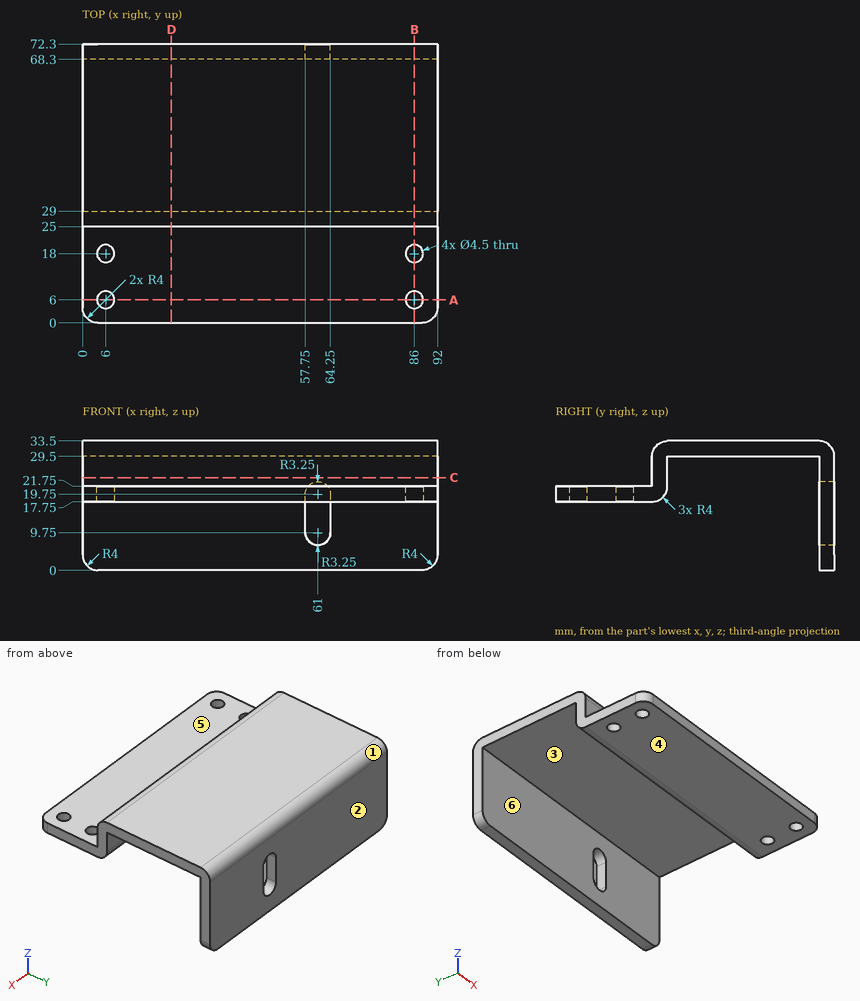
Design review of the part shown in the three views and the two pictorial views. Dimensions are in mm from the part's minimum x, y and z. A direction names the side the tool comes from. Give positions to 0.01 mm unless a question says otherwise; leave off trailing zeros. Write each loop counter-clockwise with the first axis right and the second up, starting at its lowest first coordinate (ties: lowest second). Pieces come first, ordered by that corner, then holes. Notation, with made-up numbers: M -20.5,9.25 L 27.5,9.25 A16 ccw 27.5,29.25 Z; hole C 40.25,83 d8. An arc over 180 degrees is marked long. Return JSON: item names as keys, results as strings. Group by question number.
Item 1: The part is to be moulded in two halves that separate along Z. For the marked faces 1, 2 and 3, say which applies: pulls with the +Z half, pulls with the -Z half, needs draft (parallel to the pull), parting line crosses it, or undercut.
Item 2: Clearance check with flat-ended pins moving along their axes: pin 1 Ø7 at (x, y) = (6, 18) entering from -Z; pin 2 Ø12 at (x, y) = (43, 43) entering from -Z; pin 3 Ø7.5 at (x, y) = (62.5, 11.5) entering from +Z. State where each tip first meets the part, or that it passes through.
Item 3: Tool access review of the marked faces 4, 5 and 6: name each direction out of +Z, -Z, +X, -X, +Y, -Y from which nothing blocks a thin tool from reaching the whole face with its end or side.
Item 4: Wall thickness on line 1 along Y through (x, z) = (6, 18.85) (3 decimals); line 2 along Y through (x, z) = (86, 19); line 3 along Y through (x, z) = (48, 28.5): over which ranges is each line inside the solid? List them lowest first.
Item 5: Take a section at C-C (z = 24). Give the boundary of the cut face in (x, y), plus the area to 3 significant figures.
Item 6: Take a section at A-A (y = 6). Give the boundary of the cut face in (x, z).
Item 7: Take a section at B-B (x = 86). Give the boundary of the cut face in (y, z).
Item 8: Take a section at D-D (x = 23). Give the boundary of the cut face in (y, z), plus the area to 3 significant figures.
Return value:
{
 "1": {"face 1": "pulls with the +Z half", "face 2": "needs draft", "face 3": "pulls with the -Z half"},
 "2": {"pin 1": "stops at z = 17.75", "pin 2": "stops at z = 29.5", "pin 3": "stops at z = 21.75"},
 "3": {"face 4": "-Z, +X, -X, -Y", "face 5": "+Z, +X, -X, -Y", "face 6": "-Z, +X, -X"},
 "4": {"line 1": "y = 0 to 3.75, 8.25 to 15.75, 20.25 to 27.755, 68.3 to 72.3", "line 2": "y = 0 to 3.75, 8.25 to 15.75, 20.25 to 27.9, 68.3 to 72.3", "line 3": "y = 25 to 29, 68.3 to 72.3"},
 "5": {"outline": "M 0,25 L 92,25 L 92,29 L 0,29 Z; M 0,68.3 L 92,68.3 L 92,72.3 L 0,72.3 Z", "area": "736 mm2"},
 "6": {"outline": "M 0,17.75 L 3.75,17.75 L 3.75,21.75 L 0,21.75 Z; M 8.25,17.75 L 83.75,17.75 L 83.75,21.75 L 8.25,21.75 Z; M 88.25,17.75 L 92,17.75 L 92,21.75 L 88.25,21.75 Z"},
 "7": {"outline": "M 0,17.75 L 3.75,17.75 L 3.75,21.75 L 0,21.75 Z; M 8.25,17.75 L 15.75,17.75 L 15.75,21.75 L 8.25,21.75 Z; M 20.25,17.75 L 25,17.75 A4 ccw 29,21.75 L 29,29.5 L 68.3,29.5 L 68.3,0 L 72.3,0 L 72.3,29.5 A4 ccw 68.3,33.5 L 29,33.5 A4 ccw 25,29.5 L 25,21.75 L 20.25,21.75 Z"},
 "8": {"outline": "M 0,17.75 L 25,17.75 A4 ccw 29,21.75 L 29,29.5 L 68.3,29.5 L 68.3,0 L 72.3,0 L 72.3,29.5 A4 ccw 68.3,33.5 L 29,33.5 A4 ccw 25,29.5 L 25,21.75 L 0,21.75 Z", "area": "444 mm2"}
}
